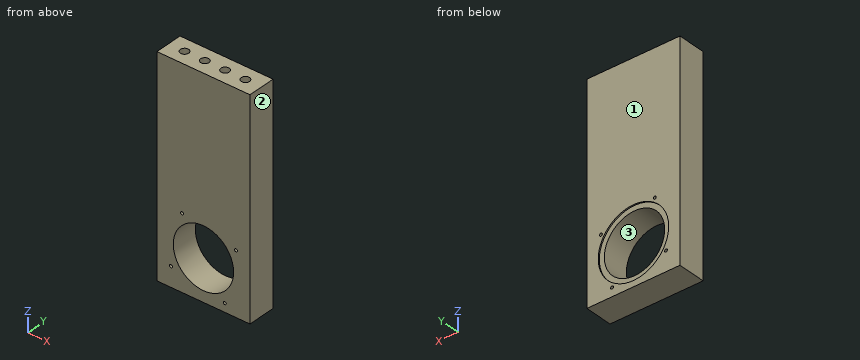
from build123d import *

# Parameters (mm, degrees)
F0_W     = 111
F0_H     = 254
F0_R     = 1.727
F0_R_2   = 36.003175
F1_DEPTH = 33.25
F2_R     = 42.045
F3_DEPTH = 1.53
F4_R     = 5
F5_DEPTH = 20


with BuildPart() as f1:
    # F0 (on Front) → F1 (new body)
    with BuildSketch(Plane.XZ):
        with Locations((-1.262473, 43.099124)):
            Rectangle(F0_W, F0_H)
        with Locations((-40.06318, -60.397701)):
            Circle(F0_R, mode=Mode.SUBTRACT)
        with Locations((-1.262473, -34.897701)):
            Circle(F0_R_2, mode=Mode.SUBTRACT)
        with Locations((-26.762473, 3.903007)):
            Circle(F0_R, mode=Mode.SUBTRACT)
        with Locations((24.237527, -73.698408)):
            Circle(F0_R, mode=Mode.SUBTRACT)
        with Locations((37.538235, -9.397701)):
            Circle(F0_R, mode=Mode.SUBTRACT)
    extrude(amount=F1_DEPTH)

    # F2 (on face) → F3 (cut)
    with BuildSketch(Plane(origin=(0, 0, 0), x_dir=(-1, 0, 0), z_dir=(0, 1, 0))):
        with Locations((1.262473, -34.897701)):
            Circle(F2_R)
    extrude(amount=-F3_DEPTH, mode=Mode.SUBTRACT)

    # F4 (on face) → F5 (cut)
    with BuildSketch(Plane.XY.offset(170.099124)):
        with Locations((-37.562473, -16.625)):
            Circle(F4_R)
        with Locations((-13.362473, -16.625)):
            Circle(F4_R)
        with Locations((10.837527, -16.625)):
            Circle(F4_R)
        with Locations((35.037527, -16.625)):
            Circle(F4_R)
    extrude(amount=-F5_DEPTH, mode=Mode.SUBTRACT)


solid = f1.part
The listing builds one solid part. Answer for the finished solid, in the listing's coordinates (mm). Face numbers are marked on the shaded views. Round coordinates to 2 decimals unless told otherwise and drop trailing zeros. Order: outer loops, then holes, each group sorted by start corner. A loop starts at its lowest first (then second) coordinate and runs counter-clockwise, first axis right, second up. Notation, with made-up numbers: (70.25, 23.25) -> (128.25, 23.25) arc R7 ccw to (128.25, 36.25) -> close; hole circle Ø2 at (7, 9.5). An arc over 180 degrees is marked (long way). Put each result on its own line as item: value.
Q1. Determine the mould class of the marked faces 1, 2 and 3 for opening direction X: pulls with the +X half, pulls with the -X half, needs draft (parallel to the pull), parting line crosses it, or undercut.
Results list:
face 1: needs draft
face 2: pulls with the +X half
face 3: undercut
Q2. Section A-A, the plane z = -32 is taken. Write down the section's boundary in (x, y).
Results list:
outline: (-56.76, -33.25) -> (-37.15, -33.25) -> (-37.15, -1.53) -> (-43.21, -1.53) -> (-43.21, 0) -> (-56.76, 0) -> close; (34.62, -33.25) -> (54.24, -33.25) -> (54.24, 0) -> (40.68, 0) -> (40.68, -1.53) -> (34.62, -1.53) -> close
Q3. This flat-tipped pin is pushed along its axis until it touches: P1, Ø3, axis at x = -26.76, z = 3.9, coming from the -Y side. Where does it stop, or does it pass through?
Results list:
P1: through
Q4. Consider line 1 along Z through (x, y) = (25, -11); line 2 along X through (y, z) = (-26.5, -34); line 3 along X through (y, z) = (-21.5, -74). Determine where each line is inside the solid, lowest interval first.
Results list:
line 1: -83.9 to -75.25, -72.15 to -59.53, -10.27 to 170.1
line 2: -56.76 to -37.25, 34.73 to 54.24
line 3: -56.76 to 22.54, 25.94 to 54.24
Q5. Section C-C, the plane y = -29 is taken. Write down the section's boundary in (x, z).
Results list:
outline: (-56.76, -83.9) -> (54.24, -83.9) -> (54.24, 170.1) -> (-56.76, 170.1) -> close; hole circle Ø3.45 at (-40.06, -60.4); hole circle Ø72.01 at (-1.26, -34.9); hole circle Ø3.45 at (-26.76, 3.9); hole circle Ø3.45 at (24.24, -73.7); hole circle Ø3.45 at (37.54, -9.4)
Q6. Section B-B, the plane x = -2 is taken. Write down the section's boundary in (y, z).
Results list:
outline: (-33.25, -83.9) -> (0, -83.9) -> (0, -76.94) -> (-1.53, -76.94) -> (-1.53, -70.89) -> (-33.25, -70.89) -> close; (-33.25, 1.1) -> (-1.53, 1.1) -> (-1.53, 7.14) -> (0, 7.14) -> (0, 170.1) -> (-33.25, 170.1) -> close
Q7. Section D-D, the plane z = 155.5 is taken. Write down the section's boundary in (x, y) (3 decimals).
Results list:
outline: (-56.762, -33.25) -> (54.238, -33.25) -> (54.238, 0) -> (-56.762, 0) -> close; hole circle Ø10 at (-37.562, -16.625); hole circle Ø10 at (-13.362, -16.625); hole circle Ø10 at (10.838, -16.625); hole circle Ø10 at (35.038, -16.625)
